Geometry check sheet. Reference: the model listing, model coordinates, mm. A direction names the side the tool comes from. Coordinates: 2 decimals unless noted, no trailing zeros. Loops run counter-clockwise (first coordinate to the right, second up) from the corner with the lowest first, then second, coordinate; pieces in that order, holes last.
from build123d import *

# Parameters (mm, degrees)
SKETCH_1_W          = 20
SKETCH_1_H          = 8
EXTRUDE_1_DEPTH     = 2
SKETCH_2_W          = 10
SKETCH_2_H          = 2.5
EXTRUDE_2_DEPTH     = 20
SKETCH_3_R          = 1.75
CUT_EXTRUDE_1_DEPTH = 20


with BuildPart() as part:
    # 草图1 → 凸台-拉伸1 (new body)
    with BuildSketch(Plane.XY):
        with Locations((10, 4)):
            Rectangle(SKETCH_1_W, SKETCH_1_H)
    extrude(amount=EXTRUDE_1_DEPTH)

    # 草图2 → 凸台-拉伸2 (add)
    with BuildSketch(Plane.XY.offset(2)):
        with Locations((10, -1.25)):
            Rectangle(SKETCH_2_W, SKETCH_2_H)
    extrude(amount=-EXTRUDE_2_DEPTH)

    # 草图3 → 切除-拉伸1 (cut)
    with BuildSketch(Plane(origin=(0, 0, 0), x_dir=(-1, 0, 0), z_dir=(0, 0, -1))):
        with Locations((-15, 4)):
            Circle(SKETCH_3_R)
        with Locations((-5, 4)):
            Circle(SKETCH_3_R)
    extrude(amount=-CUT_EXTRUDE_1_DEPTH, mode=Mode.SUBTRACT)


solid = part.part
1) Section check B-B on z = 0.25. Record the cut outline in (x, y).
Data:
outline: (0, 0) - (5, 0) - (5, -2.5) - (15, -2.5) - (15, 0) - (20, 0) - (20, 8) - (0, 8) - close; hole circle Ø3.5 at (5, 4); hole circle Ø3.5 at (15, 4)
2) Material ranges on probe 1 along Y at (x, z) = (13.75, -1); probe 2 along Z at (x, y) = (6.75, 4.5); probe 3 along X at (y, z) = (-1, -7), recorded low to high.
Data:
probe 1: y = -2.5 to 0
probe 2: z = 0 to 2
probe 3: x = 5 to 15
3) Section check D-D on y = 1.25. Record the cut outline in (x, z).
Data:
outline: (0, 0) - (20, 0) - (20, 2) - (0, 2) - close
4) Section check A-A on y = 4. Record the cut outline in (x, z), and give its area (3 significant figures).
Data:
outline: (0, 0) - (3.25, 0) - (3.25, 2) - (0, 2) - close; (6.75, 0) - (13.25, 0) - (13.25, 2) - (6.75, 2) - close; (16.75, 0) - (20, 0) - (20, 2) - (16.75, 2) - close
area: 26.0 mm2
5) Access from +Z, -Z, +X, -X, +Y, -Y to the whole of each face (thin tool, end or side, straight path). Record for faces 1 (the flat face through (17, 0, 1)), 2 (the flat face through (10, 3, 2)), 3 (the flat face through (10, 8, 1)), 4 (the flat face through (10, 4, 0)), 5 (the flat face through (2, 0, 1)).
Data:
face 1: +Z, -Z, +X, -Y
face 2: +Z, +X, -X, +Y, -Y
face 3: +Z, -Z, +X, -X, +Y
face 4: -Z, +X, -X, +Y
face 5: +Z, -Z, -X, -Y
6) Mould release check, pull along X, two halves, no side actions. Record for faces 6 (the flat face through (15, -1, -8)), 7 (the cylindrical face through (5.38, 2.29, 0.99)), 8 (the flat face through (10, 0, -9)): +X half, -X half, draft (parallel to the pull), parting line (faces both ways), or undercut.
Data:
face 6: +X half
face 7: undercut
face 8: draft
7) Depth check by flat-ended pin: pin 1 (3 mm diameter, centred on y = -1, z = -8, fed in from -X); pin 2 (1 mm diameter, centred on x = 2, z = 1, fed in from -Y); pin 3 (2.5 mm diameter, centred on x = 11, y = 5.5, fed in from -Z); pin 4 (3 mm diameter, centred on x = 5, y = 4, fed in from +Z). Enter the tip coordinate at first touch or a pass-through.
Data:
pin 1: stops at x = 5
pin 2: stops at y = 0
pin 3: stops at z = 0
pin 4: passes through
8) Section check C-C on x = 10. Record the cut outline in (y, z).
Data:
outline: (-2.5, -18) - (0, -18) - (0, 0) - (8, 0) - (8, 2) - (-2.5, 2) - close
